```python
from build123d import *

# Parameters (mm, degrees)
F0_W     = 4.5
F0_H     = 4.5
F1_DEPTH = 3
F3_DEPTH = 2
F4_SIZE  = 1


with BuildPart() as f1:
    # F0 (on Top) → F1 (new body)
    with BuildSketch(Plane.XY):
        with BuildLine():
            Line((-2.75, -3.75), (2.75, -3.75))
            ThreePointArc((2.75, -3.75), (3.457107, -3.457107), (3.75, -2.75))
            Line((3.75, -2.75), (3.75, 2.75))
            ThreePointArc((3.75, 2.75), (3.457107, 3.457107), (2.75, 3.75))
            Line((2.75, 3.75), (-2.75, 3.75))
            ThreePointArc((-2.75, 3.75), (-3.457107, 3.457107), (-3.75, 2.75))
            Line((-3.75, 2.75), (-3.75, -2.75))
            ThreePointArc((-3.75, -2.75), (-3.457107, -3.457107), (-2.75, -3.75))
        make_face()
        Rectangle(F0_W, F0_H, mode=Mode.SUBTRACT)
    extrude(amount=F1_DEPTH)

    # F2 (on face) → F3 (join)
    with BuildSketch(Plane.XY.offset(3)):
        with BuildLine():
            ThreePointArc((6, 5), (5.707107, 5.707107), (5, 6))
            Line((5, 6), (-5, 6))
            ThreePointArc((-5, 6), (-5.707107, 5.707107), (-6, 5))
            Line((-6, 5), (-6, -5))
            ThreePointArc((-6, -5), (-5.707107, -5.707107), (-5, -6))
            Line((-5, -6), (5, -6))
            ThreePointArc((5, -6), (5.707107, -5.707107), (6, -5))
            Line((6, -5), (6, 5))
        make_face()
    extrude(amount=F3_DEPTH)

    # F4
    f4_edges = [f1.edges().sort_by_distance(p)[0] for p in [
        (0, -3.75, 3),
    ]]
    chamfer(f4_edges, length=F4_SIZE)


solid = f1.part
```
Check sheet for the modelled part. Datum: model origin and axes. Units: mm. A direction names the side the tool comes from. Give positions to 0.01 mm unless a question says otherwise; leave off trailing zeros. Write each loop counter-clockwise with the first axis right and the second up, starting at its lowest first coordinate (ties: lowest second). Pieces come first, ordered by that corner, then holes. Notation, with made-up numbers: (2.5, -15) - (25.5, -15) arc R32 ccw to (25.5, 14) - close; hole circle Ø4 at (-24.5, 32). An arc over 180 degrees is marked (long way). Answer as a JSON object with one key per item and string values. Group by question number.
1) Sectioned sample at B-B (y = 1.5). Record the cut outline in (x, z), then the cut area to 3 significant figures.
2) Thickness scan on probe 1 along Y at (x, z) = (0.5, 1.35). Record the ranges inside material, lowest first. Write a range as from..to.
3) Sectioned sample at A-A (z = 2.6). Record the cut outline in (x, y), then the cut area to 3 significant figures.
4) Sectioned sample at D-D (z = 1.25). Record the cut outline in (x, y), then the cut area to 3 significant figures.
5) Depth check by flat-ended pin: P1, Ø2, axis at x = 0, y = 0, coming from the -Z side; P2, Ø0.9, axis at x = 1, z = 2, coming from the -Y side; P3, Ø2, axis at x = -1.5, z = 0.5, coming from the +Y side. Enter the tip coordinate at first touch or a pass-through.
6) Access from +Z, -Z, +X, -X, +Y, -Y to the whole of each face (thin tool, end or side, straight path). Record for faces 5 (the face through (0, -2.25, 1)), 6 (the face through (0, 3.75, 1)), 7 (the face through (3.465, 3.449, 0.986)), 8 (the face through (0, -3.75, 1)).
7) Release check for a two-part mould opening along X. For faces 1 (the face through (6, 0, 4)), 2 (the face through (-5, 0, 3)), 3 (the face through (-2.25, 0, 1)), 4 (the face through (2.25, 0, 1)) record: pulls with the +X half, pulls with the -X half, needs draft (parallel to the pull), parting line crosses it, or undercut.
8) Sectioned sample at C-C (x = 2.5). Record the cut outline in (y, z), then the cut area to 3 significant figures.
Geometry results:
{
 "1": {"outline": "(-6, 3) - (-4.75, 3) - (-3.75, 2) - (-3.75, 0) - (-2.25, 0) - (-2.25, 3) - (2.25, 3) - (2.25, 0) - (3.75, 0) - (3.75, 2) - (4.75, 3) - (6, 3) - (6, 5) - (-6, 5) - close", "area": "34.0 mm^2"},
 "2": {"probe 1": "y = -3.75..-2.25, 2.25..3.75"},
 "3": {"outline": "(-4.35, -2.75) arc R1.6 ccw to (-2.75, -4.35) - (2.75, -4.35) arc R1.6 ccw to (4.35, -2.75) - (4.35, 2.75) arc R1.6 ccw to (2.75, 4.35) - (-2.75, 4.35) arc R1.6 ccw to (-4.35, 2.75) - close; hole (-2.25, -2.25) - (2.25, -2.25) - (2.25, 2.25) - (-2.25, 2.25) - close", "area": "53.2 mm^2"},
 "4": {"outline": "(-3.75, -2.75) arc R1 ccw to (-2.75, -3.75) - (2.75, -3.75) arc R1 ccw to (3.75, -2.75) - (3.75, 2.75) arc R1 ccw to (2.75, 3.75) - (-2.75, 3.75) arc R1 ccw to (-3.75, 2.75) - close; hole (-2.25, -2.25) - (2.25, -2.25) - (2.25, 2.25) - (-2.25, 2.25) - close", "area": "35.1 mm^2"},
 "5": {"P1": "stops at z = 3", "P2": "stops at y = -4.2", "P3": "stops at y = 3.75"},
 "6": {"face 5": "-Z", "face 6": "-Z, +X, -X, +Y", "face 7": "-Z, +X, +Y", "face 8": "-Z, +X, -X, -Y"},
 "7": {"face 1": "pulls with the +X half", "face 2": "needs draft", "face 3": "undercut", "face 4": "undercut"},
 "8": {"outline": "(-6, 3) - (-4.75, 3) - (-3.75, 2) - (-3.75, 0) - (3.75, 0) - (3.75, 2) - (4.75, 3) - (6, 3) - (6, 5) - (-6, 5) - close", "area": "47.5 mm^2"}
}
